Autodesk Inventor part; units mm, degrees
ref_plane "YZ Plane" through (0, 0, 0) normal (1, 0, 0) x (0, 1, 0)
ref_plane "XZ Plane" through (0, 0, 0) normal (0, 1, 0) x (-1, 0, 0)
ref_plane "XY Plane" through (0, 0, 0) normal (0, 0, 1) x (1, 0, 0)
sketch "Sketch1" plane through (0, 0, 0) normal (0, 1, 0) x (-1, 0, 0)
  circle A0 centre (0, 0) radius 2.5
  dimension "d0" = 5
extrude "Extrusion1" add sketch "Sketch1" along normal blind 0.75
chamfer "Chamfer1" distance 0.125 angle 45 2 edges at (2.5, 0, 0) (2.5, 0.75, 0)
sketch "Sketch2" plane through (0, 0.75, 0) normal (0, 1, 0) x (1, 0, 0)
  circle A0 centre (0, 0) radius 2.25
  dimension "d6" = 4.5
extrude "Extrusion2" add sketch "Sketch2" along normal blind 30
sketch "Sketch3" plane through (0, 30.75, 0) normal (0, 1, 0) x (1, 0, 0)
  circle A0 centre (0, 0) radius 1.25
  dimension "d9" = 2.5
extrude "Extrusion3" cut sketch "Sketch3" against normal blind 5
thread "Thread1"
chamfer "Chamfer2" distance 0.125 angle 45 1 edges at (-2.25, 30.75, 0)
properties part number "Z25_Hinge_Shaft" material "Stainless Steel"
Input: part model. Units: mm. Frame: model coordinates. A direction names the side the tool comes from. Give positions to 0.01 mm unless a question says otherwise; leave off trailing zeros. Order: outer loops, then holes, each group sorted by start corner. A loop starts at its lowest first (then second) coordinate and runs counter-clockwise, first axis right, second up. Notation, with made-up numbers: (80, 62) - (139, 62) arc R21 cw to (139, 86) - close; hole circle Ø6 at (70.5, 74). An arc over 180 degrees is marked (long way). One line per item, written item: value.
1. Cut plane C-C, the plane y = 27. Output: boundary loops of the cut face in (x, z).
Determined:
outline: circle Ø4.5 at (0, 0); hole circle Ø2.5 at (0, 0)
2. Reachability of faces 1 (the face through (0, 25.75, 0)), 2 (the face through (1, 30.75, 1)) from +Z, -Z, +X, -X, +Y, -Y: full face, straight path, thin tool, end or side. Return the list, or none.
Determined:
face 1: +Y
face 2: +Z, -Z, +X, -X, +Y
3. Cut plane B-B, the plane z = 0. Output: boundary loops of the cut face in (x, y) (3 decimals), and give its area (3 significant figures).
Determined:
outline: (-2.5, 0.125) - (-2.375, 0) - (2.375, 0) - (2.5, 0.125) - (2.5, 0.625) - (2.375, 0.75) - (2.25, 0.75) - (2.25, 30.625) - (2.125, 30.75) - (1.25, 30.75) - (1.25, 25.75) - (-1.25, 25.75) - (-1.25, 30.75) - (-2.125, 30.75) - (-2.25, 30.625) - (-2.25, 0.75) - (-2.375, 0.75) - (-2.5, 0.625) - close
area: 126 mm2
4. Cut plane D-D, the plane y = 20. Output: boundary loops of the cut face in (x, z), and give its area (3 significant figures).
Determined:
outline: circle Ø4.5 at (0, 0)
area: 15.9 mm2
5. Line query: probe 1 along X at (y, z) = (28.6, 0); probe 2 along Y at (x, z) = (1, 2.05). Output: solid intervals per line, ascending.
Determined:
probe 1: -2.25 to -1.25, 1.25 to 2.25
probe 2: 0 to 0.75
6. Draft query along X for faces 3 (the face through (-0.27, 28.28, 1.22)), 4 (the face through (0, 0, 0)), 5 (the face through (0.54, 0.37, 2.44)). Return one class per face: released by +X, released by -X, zero draft, split by the parting line, or undercut.
Determined:
face 3: undercut
face 4: zero draft
face 5: split by the parting line
7. Cut plane A-A, the plane x = 0. Output: boundary loops of the cut face in (y, z) (3 decimals).
Determined:
outline: (0, -2.375) - (0.125, -2.5) - (0.625, -2.5) - (0.75, -2.375) - (0.75, -2.25) - (30.625, -2.25) - (30.75, -2.125) - (30.75, -1.25) - (25.75, -1.25) - (25.75, 1.25) - (30.75, 1.25) - (30.75, 2.125) - (30.625, 2.25) - (0.75, 2.25) - (0.75, 2.375) - (0.625, 2.5) - (0.125, 2.5) - (0, 2.375) - close
8. Pin query (flat end, axial travel): pin 1 Ø1 at (y, z) = (24, -1) entering from -X; pin 2 Ø1.4 at (x, z) = (0, 0.5) entering from +Y; pin 3 Ø2 at (x, y) = (-1.5, 3.5) entering from +Z. Return the tip coordinate at first contact, or that it passes through.
Determined:
pin 1: x = -2.19
pin 2: y = 25.75
pin 3: z = 2.19
